Job drawing, mm, ordinate dimensions from the low corner. One solid piece. Give positions to 0.01 mm unless a question says otherwise; leave off trailing zeros. Write each loop counter-clockwise with the first axis right and the second up, starting at its lowest first coordinate (ties: lowest second). Pieces come first, ordered by that corner, then holes. Notation, with made-up numbers: (-40, 68) - (-6, 68) arc R24 ccw to (-6, 81) - close; hole circle Ø6 at (6, 44). An arc over 180 degrees is marked (long way). Answer in a Markdown table with one row per item. Add a question column.
1. Drop flat-ended pins along their axis: pin 1 Ø16 at (x, z) = (11, 1885) entering from -Y; pin 2 Ø15 at (x, z) = (16, 251.5) entering from -Y; pin 3 Ø9 at (x, z) = (19.5, 998.5) entering from -Y. Give the stop position or say it passes through.
2. Probe line 1 along Z through (x, y) = (27.25, 28.5); line 2 along Z through (x, y) = (7, 26) (1 decimal); line 3 along Z through (x, y) = (10, 12.5) (1 decimal). List the from-to ranges inside material, lowest first.
3. Band-saw the part on A-A on x = 15. Write the cut outline in (y, z), plus the area to 4 significant figures.
4. Band-saw the part on B-B on z = 1455. Write the cut outline in (x, y), plus the area to 3 significant figures.
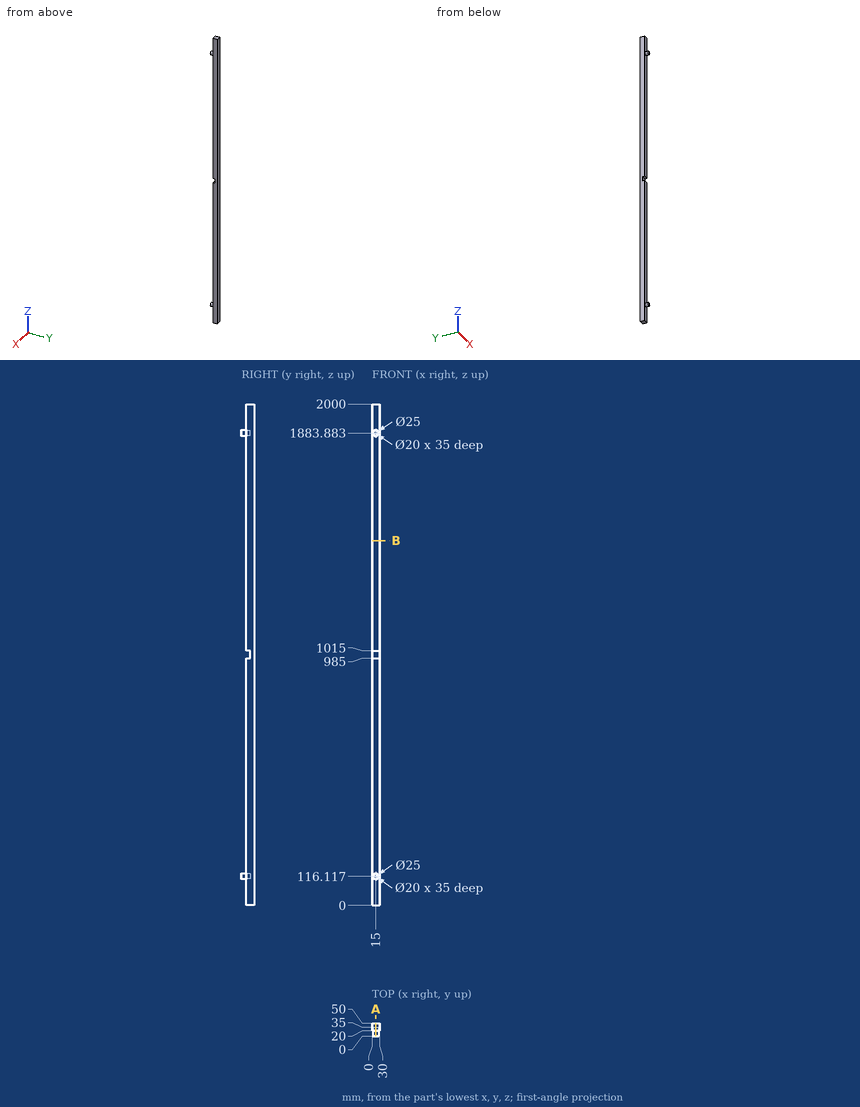
Values:
| question | item | result |
|---|---|---|
| 1 | pin 1 | stops at y = 0 |
| 1 | pin 2 | stops at y = 20 |
| 1 | pin 3 | stops at y = 35 |
| 2 | line 1 | z = 0 to 985, 1015 to 2000 |
| 2 | line 2 | z = 0 to 110.1, 122.1 to 985, 1015 to 1877.9, 1889.9 to 2000 |
| 2 | line 3 | z = 104.7 to 107.5, 124.8 to 127.6, 1872.4 to 1875.2, 1892.5 to 1895.3 |
| 3 | outline | (0, 103.62) - (20, 103.62) - (20, 0) - (50, 0) - (50, 2000) - (20, 2000) - (20, 1896.38) - (0, 1896.38) - (0, 1893.88) - (35, 1893.88) - (35, 1873.88) - (0, 1873.88) - (0, 1871.38) - (20, 1871.38) - (20, 1015) - (35, 1015) - (35, 985) - (20, 985) - (20, 128.62) - (0, 128.62) - (0, 126.12) - (35, 126.12) - (35, 106.12) - (0, 106.12) - close |
| 3 | area | 59,150 mm² |
| 4 | outline | (0, 20) - (30, 20) - (30, 50) - (0, 50) - close |
| 4 | area | 900 mm² |
